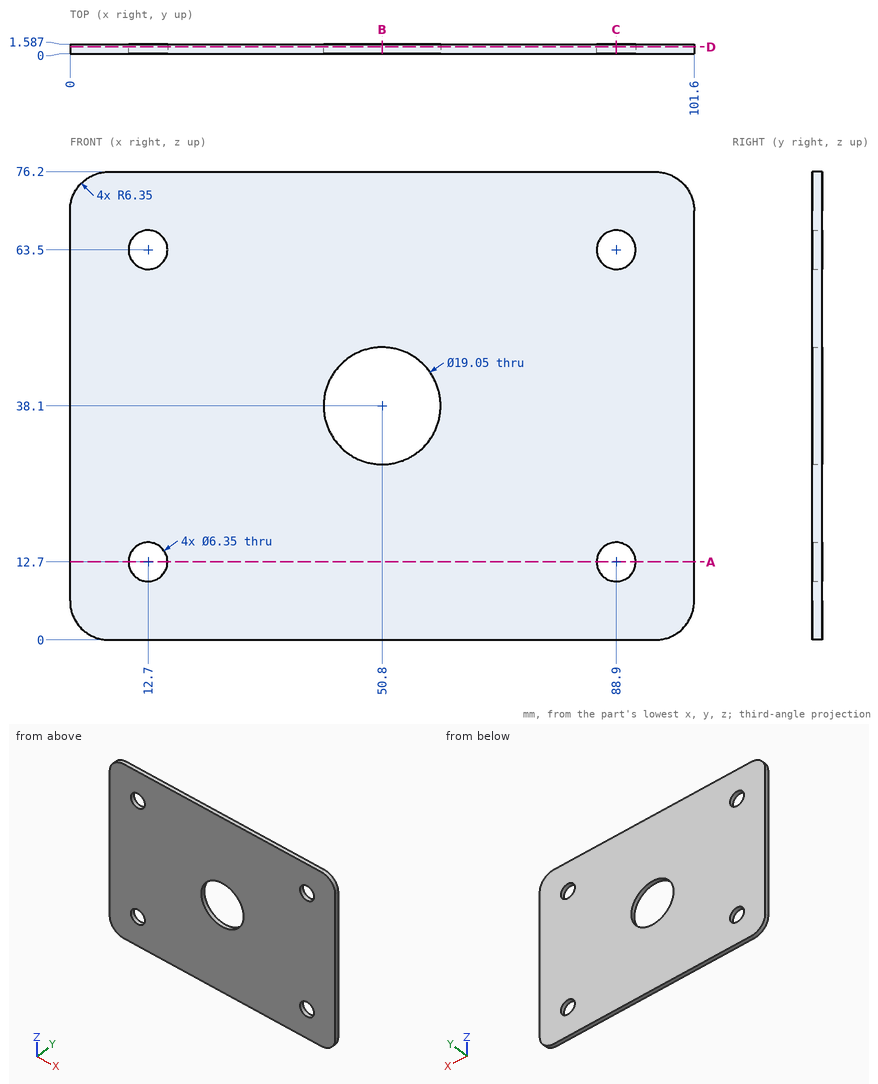
Job drawing, mm, ordinate dimensions from the low corner. One solid piece. Round coordinates to 2 decimals unless told otherwise and drop trailing zeros. Loops run counter-clockwise (first coordinate to the right, second up) from the corner with the lowest first, then second, coordinate; pieces in that order, holes last. Notation, with made-up numbers: M 25,-10 L 63,-10 A26 cw 63,10 Z; hole C 55.5,15 d5. An arc over 180 degrees is marked long. One line per question, with ' | ' between items. Start each with the question number.
Item 1: Cut at C-C, the plane x = 88.9. Write the cut outline in (y, z) (1 decimal), plus the area to 3 significant figures.
Item 2: Cut at A-A, the plane z = 12.7. Write the cut outline in (x, y) (1 decimal), plus the area to 3 significant figures.
Item 3: Wall check: line 1 (Z direction, x = 88.9, y = 0.45) (1 decimal); line 2 (X direction, y = 0.25, z = 15.5) (1 decimal); line 3 (X direction, y = 1.05, z = 38) (1 decimal). Give the ranges that are in metal, low to high.
Item 4: Cut at B-B, the plane x = 50.8. Write the cut outline in (y, z) (1 decimal).
Item 5: Cut at D-D, the plane y = 1.1. State how many separate pieces and enclosed holes the cut face has, plus the area to 3 significant figures.
Responses:
1) outline: M 0,0 L 1.6,0 L 1.6,9.5 L 0,9.5 Z; M 0,15.9 L 1.6,15.9 L 1.6,60.3 L 0,60.3 Z; M 0,66.7 L 1.6,66.7 L 1.6,76.2 L 0,76.2 Z | area: 101 mm²
2) outline: M 0,0 L 9.5,0 L 9.5,1.6 L 0,1.6 Z; M 15.9,0 L 85.7,0 L 85.7,1.6 L 15.9,1.6 Z; M 92.1,0 L 101.6,0 L 101.6,1.6 L 92.1,1.6 Z | area: 141 mm²
3) line 1: z = 0 to 9.5, 15.9 to 60.3, 66.7 to 76.2 | line 2: x = 0 to 11.2, 14.2 to 87.4, 90.4 to 101.6 | line 3: x = 0 to 41.3, 60.3 to 101.6
4) outline: M 0,0 L 1.6,0 L 1.6,28.6 L 0,28.6 Z; M 0,47.6 L 1.6,47.6 L 1.6,76.2 L 0,76.2 Z
5) separate pieces: 1 | enclosed holes: 5 | area: 7,300 mm²
